The model under review builds one solid part; all positions refer to its coordinate system, in mm. Face numbers are marked on the shaded views. A direction names the side the tool comes from. Coordinates: 2 decimals unless noted, no trailing zeros. Loops run counter-clockwise (first coordinate to the right, second up) from the corner with the lowest first, then second, coordinate; pieces in that order, holes last. Notation, with made-up numbers: M 39.25,-22 L 64.25,-22 A16 ccw 64.25,-7 Z; hole C 23,15.25 d3. An arc over 180 degrees is marked long. Use one line per item in the form item = value.
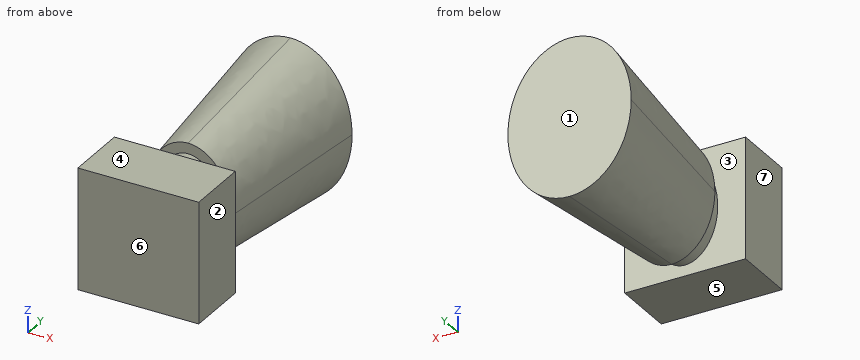
Autodesk Inventor part; units mm, degrees
ref_plane "YZ Plane" through (0, 0, 0) normal (1, 0, 0) x (0, 1, 0)
ref_plane "XZ Plane" through (0, 0, 0) normal (0, 1, 0) x (-1, 0, 0)
ref_plane "XY Plane" through (0, 0, 0) normal (0, 0, 1) x (1, 0, 0)
sketch "Sketch2" plane through (0, 0, 0) normal (0, 1, 0) x (-1, 0, 0)
  line L0 (25.7555, -11.7629) -> (11.1505, -11.7629)
  line L1 (11.1505, -11.7629) -> (11.1505, -26.3679)
  line L2 (11.1505, -26.3679) -> (25.7555, -26.3679)
  line L3 (25.7555, -26.3679) -> (25.7555, -11.7629)
  point P0 (0, 0)
  dimension "d0" = 14.605
  dimension "d1" = 14.605
extrude "Extrusion1" add sketch "Sketch2" along normal blind 7.62
sketch "Sketch3" plane through (0, 7.62, 0) normal (0, 1, 0) x (1, 0, 0)
  ellipse E0 centre (-18.453, 19.0654) end of major axis (-18.453, 25.0598) minor radius 3.937
  ellipse E1 centre (-18.453, 19.0654) end of major axis (-18.453, 26.3298) minor radius 5.207
  point P0 (0, 0)
  dimension "d13" = 5.9944
  dimension "d14" = 3.937
  dimension "d15" = 5.207
  dimension "d16" = 7.2644
extrude "Extrusion3" add sketch "Sketch3" along normal blind 2.794 contours E0
sketch "Sketch6" plane through (0, 10.414, 0) normal (0, 1, 0) x (1, 0, 0)
  ellipse E0 centre (-18.453, 19.0654) end of major axis (-18.453, 26.3298) minor radius 5.207
  ellipse E1 centre (-18.453, 19.0654) end of major axis (-18.453, 13.071) minor radius 3.937
  ellipse E2 centre (-18.453, 19.0654) end of major axis (-18.453, 26.3298) minor radius 5.207
  point P0 (0, 0)
extrude "Extrusion4" add sketch "Sketch6" along normal blind 21.336 draft 6 contours E0 | E1
ref_plane "Work Plane2" through (-18.453, 0, -11.7629) normal (1, 0, 0) x (0, 0, -1)
sketch "Sketch9" plane through (-18.453, 0, -11.7629) normal (1, 0, 0) x (0, 0, -1)
  arc A0 (23.2608, 28.3606) -> (-8.4979, 28.3606) centre (7.3815, 6.1892) ccw
  line L0 (-8.4979, 28.3606) -> (23.2608, 28.3606)
  line L1 (23.2608, 28.3606) -> (14.605, 0)
  line L2 (14.605, 0) -> (0, 0)
  line L3 (14.605, 0) -> (0, 0)
  line L4 (0, 0) -> (-8.4979, 28.3606)
  point P0 (-11.7629, 0)
properties part number "MalePassengerTL"
1. Insertion check: P1, Ø8.5, axis at x = -21.5, y = 3, coming from the +Z side; P2, Ø2, axis at y = 20, z = -16.5, coming from the +X side; P3, Ø1.5, axis at y = 24.5, z = -15, coming from the +X side. Each pin has a flat end and moves straight along its axis. Give the tip position at first contact, or say it passes through.
Response values:
P1 = -11.76
P2 = -12.32
P3 = -12.24
2. Add section A-A (y = 3.5). State the section outline as (x, z) points.
Response values:
outline = M -25.76,-26.37 L -11.15,-26.37 L -11.15,-11.76 L -25.76,-11.76 Z
3. Wall thickness on line 1 along Y through (x, z) = (-14.75, -16.5); line 2 along X through (y, z) = (2, -16.5); line 3 along Y through (x, z) = (-12.5, -13): over which ranges is each line inside the solid? List them lowest first. Write a range as from..to.
Response values:
line_1 = 0..7.62, 10.41..31.75
line_2 = -25.76..-11.15
line_3 = 0..7.62
4. The part is to be moulded in two halves that separate along Y. For the marked faces 1, 2 and 3, say which applies: pulls with the +Y half, pulls with the -Y half, needs draft (parallel to the pull), parting line crosses it, or undercut.
Response values:
face_1 = pulls with the +Y half
face_2 = needs draft
face_3 = undercut
5. Machinability: for the marked faces 4, 5, 6 and 7, which of the approach directions +Z, -Z, +X, -X, +Y, -Y give a long, thin tool a straight path to every point of the face, cutting with its end or side? Answer none if there is none.
Response values:
face_4 = +Z, +X, -X, -Y
face_5 = -Z, +X, -X, -Y
face_6 = +Z, -Z, +X, -X, -Y
face_7 = +Z, -Z, -X, -Y
